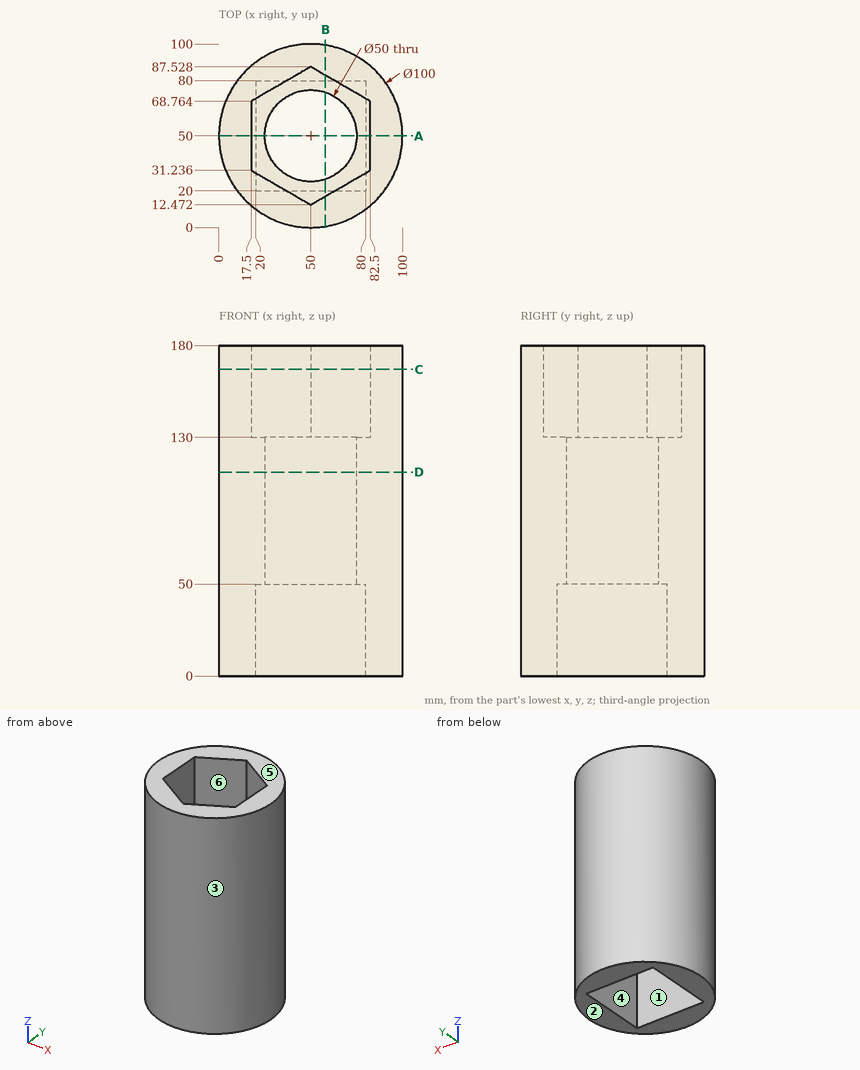
Answer from the drawing. Dimensions are ordinates in mm from the lowest x, y and z of the part. A direction names the side the tool comes from. Coordinates: 2 decimals unless noted, no trailing zeros. Loops run counter-clockwise (first coordinate to the right, second up) from the corner with the lowest first, then second, coordinate; pieces in that order, holes last. Notation, with made-up numbers: (16.25, 74) -> (46.25, 74) arc R22 ccw to (46.25, 109) -> close; hole circle Ø1 at (53, 36.5). An arc over 180 degrees is marked (long way). Answer in a Markdown table with one row per item.
Item 1: For a pull along Y with two mould halves and no side action, classify the marked faces 1, 2 and 3 as released by +Y, released by -Y, zero draft, split by the parting line, or undercut.
Returned:
| item | result |
|---|---|
| face 1 | undercut |
| face 2 | zero draft |
| face 3 | split by the parting line |
Item 2: A cutting plane is placed at C-C on z = 167. Determine the outline of the cut face in (x, y), plus the area to 4 significant figures.
Returned:
| item | result |
|---|---|
| outline | circle Ø100 at (50, 50); hole (17.5, 31.24) -> (50, 12.47) -> (82.5, 31.24) -> (82.5, 68.76) -> (50, 87.53) -> (17.5, 68.76) -> close |
| area | 4,195 mm^2 |
Item 3: For the marked faces 4, 5 and 6, determine the directions among +Z, -Z, +X, -X, +Y, -Y from which every point of the face is accessible in a straight line to the end or side of a thin tool.
Returned:
| item | result |
|---|---|
| face 4 | -Z |
| face 5 | +Z, +X, -X, +Y, -Y |
| face 6 | +Z |
Item 4: Each of these flat-tipped pins is pushed along its axis until it touches: P1, Ø1, axis at x = 33, y = 21, coming from the -Z side; P2, Ø25, axis at x = 57.5, z = 26, coming from the +Y side; P3, Ø4, axis at y = 25.5, z = 86, coming from the -X side. Where does it stop, or does it pass through?
Returned:
| item | result |
|---|---|
| P1 | stops at z = 50 |
| P2 | stops at y = 100 |
| P3 | stops at x = 5.35 |
Item 5: A cutting plane is placed at A-A on y = 50. Determine the outline of the cut face in (x, z).
Returned:
| item | result |
|---|---|
| outline | (0, 0) -> (20, 0) -> (20, 50) -> (25, 50) -> (25, 130) -> (17.5, 130) -> (17.5, 180) -> (0, 180) -> close; (75, 50) -> (80, 50) -> (80, 0) -> (100, 0) -> (100, 180) -> (82.5, 180) -> (82.5, 130) -> (75, 130) -> close |
Item 6: A cutting plane is placed at D-D on z = 111. Determine the outline of the cut face in (x, y), plus the area to 3 significant figures.
Returned:
| item | result |
|---|---|
| outline | circle Ø100 at (50, 50); hole circle Ø50 at (50, 50) |
| area | 5,890 mm^2 |
Item 7: Straight lines are drawn through the part: line 1 along Y through (x, z) = (50, 110); line 2 along Z through (x, y) = (76.5, 78); line 3 along X through (y, z) = (31, 143.5). For each, find the intervals that lie inside material, in ascending order. Write a range as [from, to].
Returned:
| item | result |
|---|---|
| line 1 | y = [0, 25], [75, 100] |
| line 2 | z = [50, 180] |
| line 3 | x = [3.75, 17.91], [82.09, 96.25] |
Item 8: A cutting plane is placed at B-B on x = 58. Determine the outline of the cut face in (y, z) (1 decimal), plus the area to 3 significant figures.
Returned:
| item | result |
|---|---|
| outline | (0.6, 0) -> (20, 0) -> (20, 50) -> (26.3, 50) -> (26.3, 130) -> (17.1, 130) -> (17.1, 180) -> (0.6, 180) -> close; (73.7, 50) -> (80, 50) -> (80, 0) -> (99.4, 0) -> (99.4, 180) -> (82.9, 180) -> (82.9, 130) -> (73.7, 130) -> close |
| area | 7,690 mm^2 |
